Part model, mm, in its own coordinate system. A direction names the side the tool comes from. Round coordinates to 2 decimals unless told otherwise and drop trailing zeros. Order: outer loops, then holes, each group sorted by start corner. A loop starts at its lowest first (then second) coordinate and runs counter-clockwise, first axis right, second up. Notation, with made-up numbers: (28.5, 55.25) -> (82.5, 55.25) arc R23 cw to (82.5, 90.25) -> close; hole circle Ø3 at (59.25, 8.25). An arc over 180 degrees is marked (long way). Answer as a JSON object with one key per item and string values. Group by question number.
Autodesk Inventor part; units mm, degrees
ref_plane "YZ Plane" through (0, 0, 0) normal (1, 0, 0) x (0, 1, 0)
ref_plane "XZ Plane" through (0, 0, 0) normal (0, 1, 0) x (-1, 0, 0)
ref_plane "XY Plane" through (0, 0, 0) normal (0, 0, 1) x (1, 0, 0)
sketch "Sketch1" plane through (0, 0, 0) normal (1, 0, 0) x (0, 1, 0)
  line L0 (159, 32) -> (159, -32)
  line L1 (159, -32) -> (89, -32)
  line L2 (89, -32) -> (89, -60)
  line L3 (89, -60) -> (-89, -60)
  line L4 (159, 32) -> (147, 32)
  line L5 (147, 32) -> (147, 67)
  line L6 (147, 67) -> (-147, 67)
  line L7 (-147, 67) -> (-147, 32)
  line L8 (-147, 32) -> (-159, 32)
  line L9 (-159, 32) -> (-159, -32)
  line L10 (-159, -32) -> (-89, -32)
  line L11 (-89, -32) -> (-89, -60)
  point P0 (0, 0)
  point P1 (159, 0)
  point P2 (0, 67)
  dimension "d0" = 64
  dimension "d1" = 70
  dimension "d2" = 178
  dimension "d3" = 28
  dimension "d4" = 12
  dimension "d5" = 35
  dimension "d6" = 12
  dimension "d7" = 64
  dimension "d8" = 70
  dimension "d9" = 35
extrude "Extrusion1" add sketch "Sketch1" along normal blind 20
properties part number "battlebotspinner20mmplate"
Q1. Which spindle directions (+Z, -Z, +X, -X, +Y, -Y) get a long thin tool onto all of the face, cutting with end or side? Do faces 1 (the flat face through (10, 89, -46)), 2 (the flat face through (10, -124, -32)), 3 (the flat face through (10, -147, 50)), 4 (the flat face through (10, 153, 32)), 5 (the flat face through (10, 2, 67)). Say none if no direction does.
Q2. Band-saw the part on A-A (x = 11.5). List the corners of the cut face in (y, z), plus the area to 3 significant figures.
Q3. Band-saw the part on C-C (y = 106). List the corners of the cut face in (x, z), plus the area to 3 significant figures.
Q4. Drop flat-ended pins along their axis: pin 1 Ø4 at (x, y) = (10.5, -102.5) entering from -Z; pin 2 Ø2 at (x, z) = (11, 45.5) entering from -Y; pin 3 Ø1.5 at (x, z) = (15.5, 43) entering from +Y. Give the stop position or say it passes through.
Q5. Wall check: line 1 (Y direction, x = 12.25, z = 46.5); line 2 (Z direction, x = 6.5, y = -125). Give the ranges that are in metal, low to high. Write a range as [from, to].
Q6. Band-saw the part on B-B (z = 42). List the corners of the cut face in (x, y), plus the area to 3 significant figures.
Completed:
{
 "1": {"face 1": "-Z, +X, -X, +Y", "face 2": "-Z, +X, -X, -Y", "face 3": "+Z, +X, -X, -Y", "face 4": "+Z, +X, -X, +Y", "face 5": "+Z, +X, -X, +Y, -Y"},
 "2": {"outline": "(-159, -32) -> (-89, -32) -> (-89, -60) -> (89, -60) -> (89, -32) -> (159, -32) -> (159, 32) -> (147, 32) -> (147, 67) -> (-147, 67) -> (-147, 32) -> (-159, 32) -> close", "area": "35,600 mm2"},
 "3": {"outline": "(0, -32) -> (20, -32) -> (20, 67) -> (0, 67) -> close", "area": "1,980 mm2"},
 "4": {"pin 1": "z = -32", "pin 2": "y = -147", "pin 3": "y = 147"},
 "5": {"line 1": "[-147, 147]", "line 2": "[-32, 67]"},
 "6": {"outline": "(0, -147) -> (20, -147) -> (20, 147) -> (0, 147) -> close", "area": "5,880 mm2"}
}
